Geometry: final body of the model. Coordinates: model frame, mm. Face numbers are marked on the shaded views. A direction names the side the tool comes from. Give positions to 0.01 mm unless a question says otherwise; leave off trailing zeros. Loops run counter-clockwise (first coordinate to the right, second up) from the corner with the lowest first, then second, coordinate; pieces in that order, holes last.
```python
from build123d import *

# Parameters (mm, degrees)
SKETCH1_R           = 1.9
BOSS_EXTRUDE1_DEPTH = 1.6
SKETCH2_W           = 10.6
SKETCH2_H           = 20
BOSS_EXTRUDE2_DEPTH = 3
SKETCH4_R           = 1
CUT_EXTRUDE1_DEPTH  = 3


with BuildPart() as part:
    # Sketch1 → Boss-Extrude1 (new body)
    with BuildSketch(Plane.XY):
        Polygon((-7.5, 6.464954653), (-5, 8.65), (10, 8.65), (10, -11.35), (-5, -11.35), (-7.5, -9.164954653), align=None)
        with Locations((-4.5, -1.35)):
            Circle(SKETCH1_R, mode=Mode.SUBTRACT)
    extrude(amount=BOSS_EXTRUDE1_DEPTH)

    # Sketch2 → Boss-Extrude2 (add)
    with BuildSketch(Plane.XY.offset(1.6)):
        with Locations((4.7, -1.35)):
            Rectangle(SKETCH2_W, SKETCH2_H)
    extrude(amount=BOSS_EXTRUDE2_DEPTH)

    # Sketch4 → Cut-Extrude1 (cut)
    with BuildSketch(Plane.XY.offset(4.6)):
        with Locations((4.7, -11.35)):
            Circle(SKETCH4_R)
        with Locations((4.7, 8.65)):
            Circle(SKETCH4_R)
    extrude(amount=-CUT_EXTRUDE1_DEPTH, mode=Mode.SUBTRACT)


solid = part.part
```
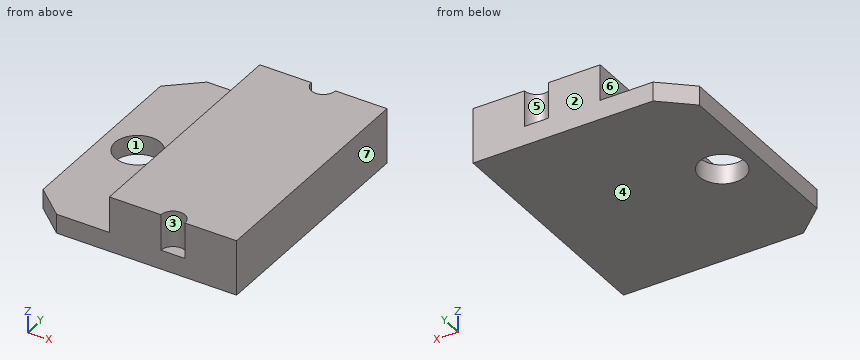
Q1. Mould query, pull axis Y, two halves, no side actions, for the marked faces 1, 2, 3 and 4. Classes: +Y half, -Y half, draft (parallel to the pull), parting line (faces both ways), or undercut.
Q2. Pin query (flat end, axial travel): pin 1 Ø2 at (y, z) = (4, 4) entering from -X; pin 2 Ø2 at (x, y) = (-2, -4.5) entering from +Z. Return the tip coordinate at first contact, or that it passes through.
Q3. Reachability of the marked faces 5, 6 and 7 from +Z, -Z, +X, -X, +Y, -Y: full face, straight path, thin tool, end or side. Return the list, or none.
Q4. Section query D-D, the plane x = 4.7. Return loops of the section in (y, z), and give its area (3 significant figures).
Q5. Section query A-A, the plane x = -4.5. Return loops of the section in (y, z), and give its area (3 significant figures).
Q6. Section query C-C, the plane z = 0.6. Return loops of the section in (x, y).
Q7. Material intervals for probe 1 along Y at (x, z) = (-4.5, 0.55); probe 2 along Z at (x, y) = (-5, 3.25); probe 3 along X at (y, z) = (-2, 3.75), sorted ascending.
Q8. Section query B-B, the plane y = -1.35. Return loops of the section in (x, z).
Resolved:
1. face 1: undercut
1. face 2: +Y half
1. face 3: -Y half
1. face 4: draft
2. pin 1: stops at x = -0.6
2. pin 2: stops at z = 1.6
3. face 5: +Z, +Y
3. face 6: +Z, -X, +Y, -Y
3. face 7: +Z, -Z, +X, +Y, -Y
4. outline: (-11.35, 0) - (8.65, 0) - (8.65, 1.6) - (7.65, 1.6) - (7.65, 4.6) - (-10.35, 4.6) - (-10.35, 1.6) - (-11.35, 1.6) - close
4. area: 86.0 mm2
5. outline: (-11.35, 0) - (-3.25, 0) - (-3.25, 1.6) - (-11.35, 1.6) - close; (0.55, 0) - (8.65, 0) - (8.65, 1.6) - (0.55, 1.6) - close
5. area: 25.9 mm2
6. outline: (-7.5, -9.16) - (-5, -11.35) - (10, -11.35) - (10, 8.65) - (-5, 8.65) - (-7.5, 6.46) - close; hole circle Ø3.8 at (-4.5, -1.35)
7. probe 1: y = -11.35 to -3.25, 0.55 to 8.65
7. probe 2: z = 0 to 1.6
7. probe 3: x = -0.6 to 10
8. outline: (-7.5, 0) - (-6.4, 0) - (-6.4, 1.6) - (-7.5, 1.6) - close; (-2.6, 0) - (10, 0) - (10, 4.6) - (-0.6, 4.6) - (-0.6, 1.6) - (-2.6, 1.6) - close
